Could you check a few things on this drawing? It's one solid part, dimensions in mm from its lowest x, y, z. A direction names the side the tool comes from. Coordinates: 2 decimals unless noted, no trailing zeros. Write each loop counter-clockwise with the first axis right and the second up, starting at its lowest first coordinate (ties: lowest second). Pieces come first, ordered by that corner, then holes.
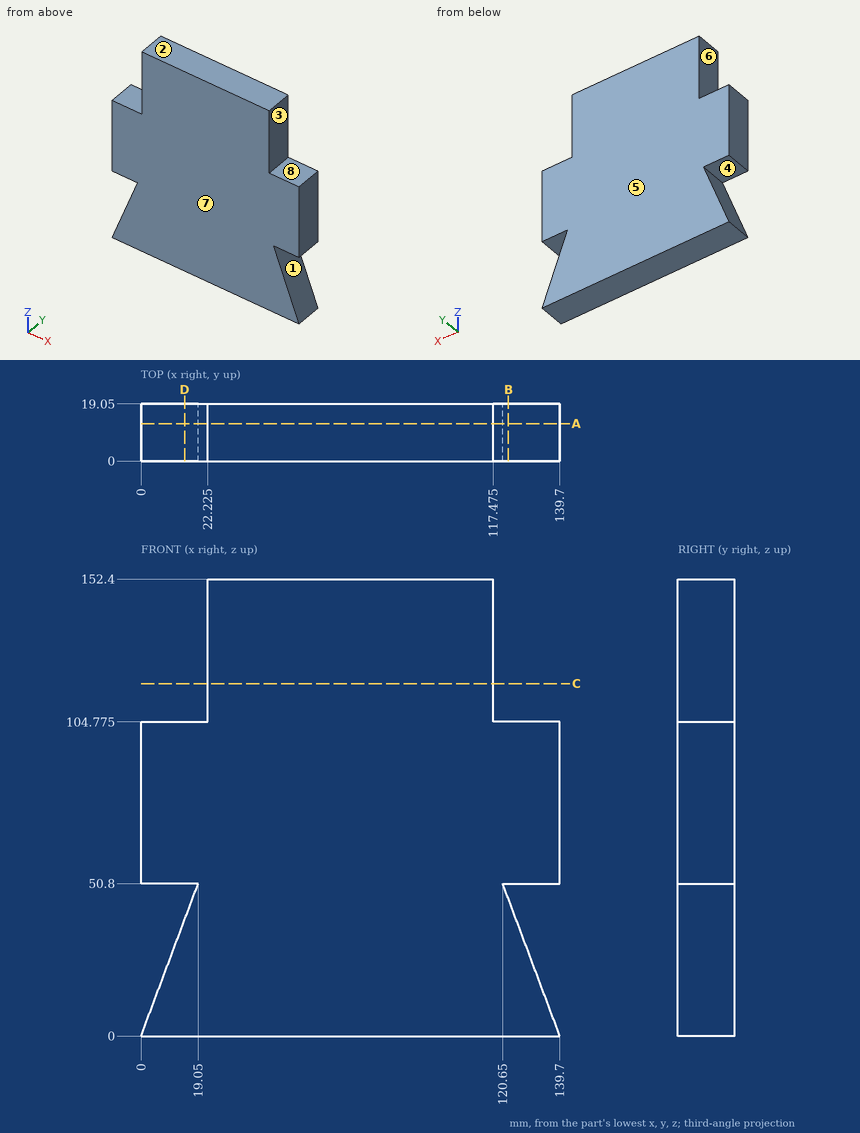
1) Imagine slicing it at A-A on y = 12.5. Please give me the cut outline in (x, z) (3 decimals).
Values follow:
outline: (0, 0) - (139.7, 0) - (120.65, 50.8) - (139.7, 50.8) - (139.7, 104.775) - (117.475, 104.775) - (117.475, 152.4) - (22.225, 152.4) - (22.225, 104.775) - (0, 104.775) - (0, 50.8) - (19.05, 50.8) - close
2) Imagine slicing it at D-D on x = 14.5. Please give me the cut outline in (y, z) (3 decimals).
Values follow:
outline: (0, 0) - (19.05, 0) - (19.05, 38.667) - (0, 38.667) - close; (0, 50.8) - (19.05, 50.8) - (19.05, 104.775) - (0, 104.775) - close
3) We'd pull the mould along Z, two halves only. Please class the marked faces 1, 2 and 3: pulls with the +Z half, pulls with the -Z half, needs draft (parallel to the pull), parting line crosses it, or undercut.
Values follow:
face 1: undercut
face 2: pulls with the +Z half
face 3: needs draft
4) Imagine slicing it at C-C on z = 117.5. Please give me the cut outline in (x, y) (3 decimals).
Values follow:
outline: (22.225, 0) - (117.475, 0) - (117.475, 19.05) - (22.225, 19.05) - close
5) Imagine slicing it at B-B on x = 122.5. Please give me the cut outline in (y, z) (3 decimals), then the cut area to 3 significant figures.
Values follow:
outline: (0, 0) - (19.05, 0) - (19.05, 45.867) - (0, 45.867) - close; (0, 50.8) - (19.05, 50.8) - (19.05, 104.775) - (0, 104.775) - close
area: 1,900 mm2
6) On a 3-axis mill with a long thin cutter (end or side, diameter ignored), from which of +Z, -Z, +X, -X, +Y, -Y can I reach the whole of each face in a straight line? I mean the marked faces 4, 5, 6, 7 and 8. Say none if no direction works.
Values follow:
face 4: -X, +Y, -Y
face 5: +Z, -Z, +X, -X, +Y
face 6: +Z, -X, +Y, -Y
face 7: +Z, -Z, +X, -X, -Y
face 8: +Z, +X, +Y, -Y
7) I need wall thicknesses on probe 1 along X at (y, z) = (12.75, 125) (3 decimals); probe 2 along X at (y, z) = (13.75, 35) (3 decimals). Which ranges of each line are inside material? Lowest first, please.
Values follow:
probe 1: x = 22.225 to 117.475
probe 2: x = 13.125 to 126.575
8) Will these pins go through, and if not, where does the flat tip stop? pin 1 (3 mm diameter, centred on x = 16.5, y = 5, fed in from +Z) (3 decimals); pin 2 (1.5 mm diameter, centred on y = 12, z = 132.5, fed in from +X) (3 decimals).
Values follow:
pin 1: stops at z = 104.775
pin 2: stops at x = 117.475
